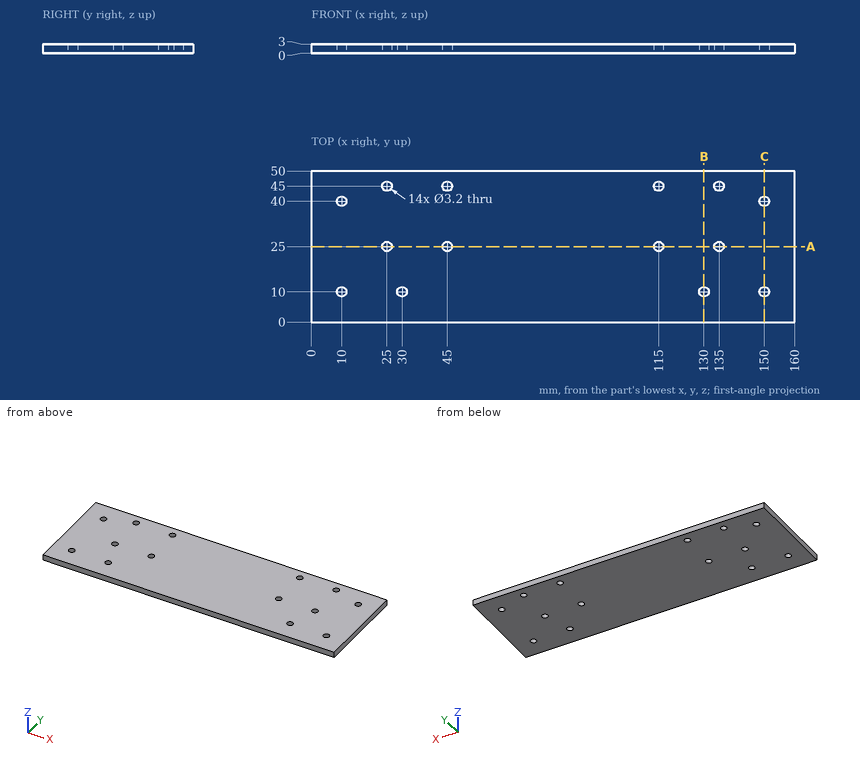
Source: three-view drawing plus pictorial views. Frame: mm from the lowest corner of the part. Round coordinates to 2 decimals unless told otherwise and drop trailing zeros. Loops run counter-clockwise (first coordinate to the right, second up) from the corner with the lowest first, then second, coordinate; pieces in that order, holes last.
Q1. Material intervals for L1, parallel to Y at x = 115, z = 1.3; L2, parallel to X at y = 45, z = 1.7; L3, parallel to X at y = 40, z = 2.7, sorted ascending.
Q2. Section B-B on x = 130. Return loops of the section in (y, z).
Q3. Section A-A on y = 25. Return loops of the section in (x, z), plus the area to 3 significant figures.
Q4. Section C-C on x = 150. Return loops of the section in (y, z), plus the area to 3 significant figures.
Q5. Pin query (flat end, axial travel): P1, Ø3.5, axis at x = 150, y = 40, coming from the +Z side. Return the tip coordinate at first contact, or that it passes through.
Evaluation:
1. L1: y = 0 to 23.4, 26.6 to 43.4, 46.6 to 50
1. L2: x = 0 to 23.4, 26.6 to 43.4, 46.6 to 113.4, 116.6 to 133.4, 136.6 to 160
1. L3: x = 0 to 8.4, 11.6 to 148.4, 151.6 to 160
2. outline: (0, 0) - (8.4, 0) - (8.4, 3) - (0, 3) - close; (11.6, 0) - (50, 0) - (50, 3) - (11.6, 3) - close
3. outline: (0, 0) - (23.4, 0) - (23.4, 3) - (0, 3) - close; (26.6, 0) - (43.4, 0) - (43.4, 3) - (26.6, 3) - close; (46.6, 0) - (113.4, 0) - (113.4, 3) - (46.6, 3) - close; (116.6, 0) - (133.4, 0) - (133.4, 3) - (116.6, 3) - close; (136.6, 0) - (160, 0) - (160, 3) - (136.6, 3) - close
3. area: 442 mm2
4. outline: (0, 0) - (8.4, 0) - (8.4, 3) - (0, 3) - close; (11.6, 0) - (38.4, 0) - (38.4, 3) - (11.6, 3) - close; (41.6, 0) - (50, 0) - (50, 3) - (41.6, 3) - close
4. area: 131 mm2
5. P1: stops at z = 3
